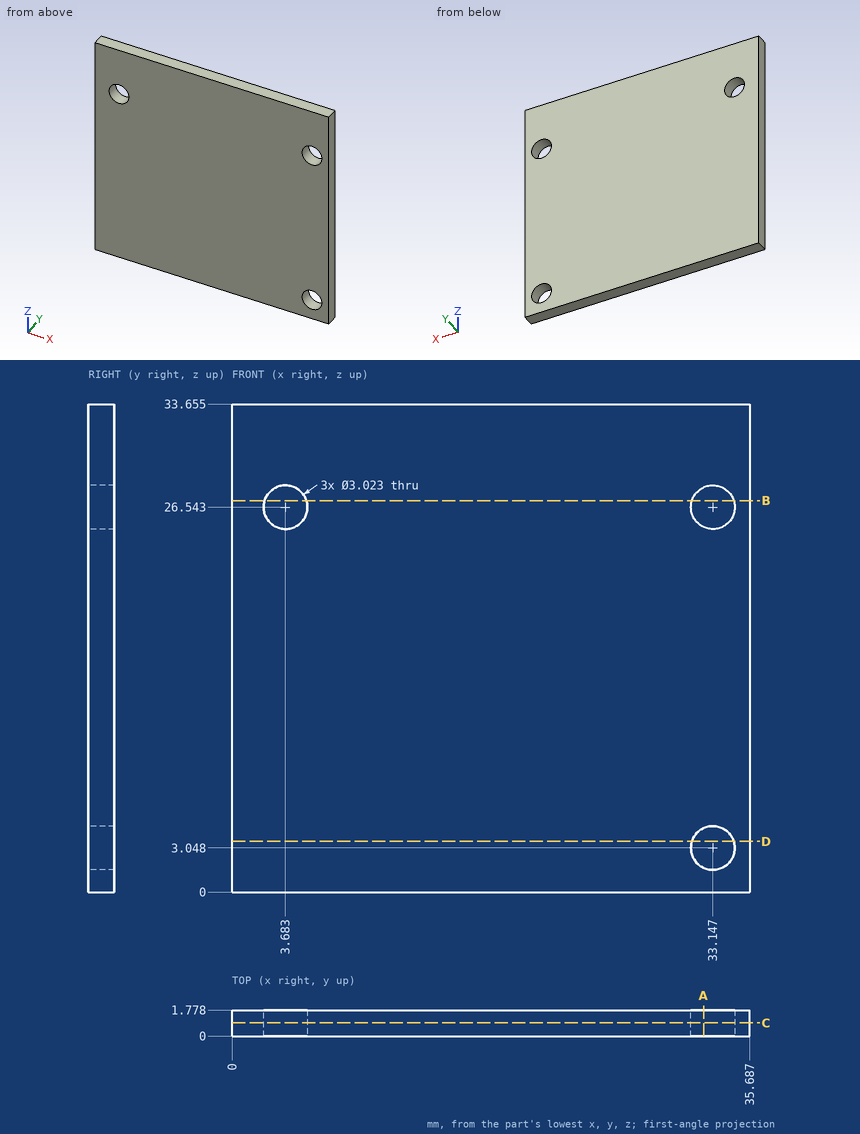
Could you check a few things on this drawing? It's one solid part, dimensions in mm from its lowest x, y, z. Round coordinates to 2 decimals unless told otherwise and drop trailing zeros. Order: outer loops, then holes, each group sorted by start corner. A loop starts at its lowest first (then second) coordinate and runs counter-clockwise, first axis right, second up. Notation, with made-up numbers: M 72,72 L 77,72 A17 ccw 77,96 Z; hole C 12.5,-22 d9. An arc over 180 degrees is marked long. Return JSON: item names as keys, results as strings. Group by question number.
1. If we section it at D-D on z = 3.5: List the corners of the cut face in (x, y) for me (1 decimal).
2. If we section it at B-B on z = 27: List the corners of the cut face in (x, y) for me.
3. If we section it at C-C on y = 0.9: List the corners of the cut face in (x, z) for me (1 decimal).
4. Please list where these lines run through material, in increasing order: probe 1 along Z at (x, y) = (34.5, 0.15) (1 decimal); probe 2 along X at (y, z) = (1, 25.5) (1 decimal); probe 3 along Z at (x, y) = (34, 1.4) (1 decimal).
5. I'm going to push a flat-ended pin straight in: pin 1 Ø2.5 at (x, z) = (33.147, 26.543) entering from -Y. Where does the tip first touch, or does it pass through?
6. If we section it at A-A on x = 32.5: List the corners of the cut face in (y, z) for me (1 decimal).
Reply:
{
 "1": {"outline": "M 0,0 L 31.7,0 L 31.7,1.8 L 0,1.8 Z; M 34.6,0 L 35.7,0 L 35.7,1.8 L 34.6,1.8 Z"},
 "2": {"outline": "M 0,0 L 2.24,0 L 2.24,1.78 L 0,1.78 Z; M 5.12,0 L 31.71,0 L 31.71,1.78 L 5.12,1.78 Z; M 34.59,0 L 35.69,0 L 35.69,1.78 L 34.59,1.78 Z"},
 "3": {"outline": "M 0,0 L 35.7,0 L 35.7,33.7 L 0,33.7 Z; hole C 3.7,26.5 d3; hole C 33.1,3 d3; hole C 33.1,26.5 d3"},
 "4": {"probe 1": "0 to 2.4, 3.7 to 25.9, 27.2 to 33.7", "probe 2": "0 to 2.6, 4.8 to 32.1, 34.2 to 35.7", "probe 3": "0 to 1.8, 4.3 to 25.3, 27.8 to 33.7"},
 "5": {"pin 1": "through"},
 "6": {"outline": "M 0,0 L 1.8,0 L 1.8,1.7 L 0,1.7 Z; M 0,4.4 L 1.8,4.4 L 1.8,25.2 L 0,25.2 Z; M 0,27.9 L 1.8,27.9 L 1.8,33.7 L 0,33.7 Z"}
}
